Autodesk Inventor part; units mm, degrees
ref_plane "YZ Plane" through (0, 0, 0) normal (1, 0, 0) x (0, 1, 0)
ref_plane "XZ Plane" through (0, 0, 0) normal (0, 1, 0) x (-1, 0, 0)
ref_plane "XY Plane" through (0, 0, 0) normal (0, 0, 1) x (1, 0, 0)
sketch "Sketch1" plane through (0, 0, 0) normal (0, 1, 0) x (-1, 0, 0)
  line L0 (0, 0) -> (0, 12.8)
  line L1 (0, 12.8) -> (-2, 12.8)
  line L2 (-2, 12.8) -> (-2, 7.8)
  line L3 (-2, 7.8) -> (-3, 7.8)
  line L4 (-3, 7.8) -> (-3, 2.8)
  line L5 (-3, 2.8) -> (-5, 2.8)
  line L6 (-5, 2.8) -> (-5, 0)
  line L7 (-5, 0) -> (0, 0)
  dimension "d0" = 10
  dimension "d1" = 6
  dimension "d2" = 4
  dimension "d3" = 5
  dimension "d4" = 5
  dimension "d5" = 2.8
revolve "Revolution1" add sketch "Sketch1" angle 360 about axis through (0, 0, 0) along (0, 0, 1)
thread "Thread1"
sketch "Sketch2" plane through (0, 0, 0) normal (0, 0, -1) x (-1, 0, 0)
  line L0 (0, 1.4434) -> (1.25, 0.7217)
  line L1 (1.25, 0.7217) -> (1.25, -0.7217)
  line L2 (1.25, -0.7217) -> (0, -1.4434)
  line L3 (0, -1.4434) -> (-1.25, -0.7217)
  line L4 (-1.25, -0.7217) -> (-1.25, 0.7217)
  line L5 (-1.25, 0.7217) -> (0, 1.4434)
  point P0 (0, 0)
  point P1 (0, 0)
  dimension "d9" = 2.5
extrude "Extrusion1" cut sketch "Sketch2" against normal blind 2
chamfer "Chamfer1" distance 0.43 angle 45 1 edges at (-2, 0, 12.8)
properties part number "DBSY4-5-5" material "Stainless Steel AISI 304"
Could you check a few things on this model? Use its own coordinates, in mm. A direction names the side the tool comes from. Give positions to 0.01 mm unless a question says otherwise; leave off trailing zeros. Order: outer loops, then holes, each group sorted by start corner. A loop starts at its lowest first (then second) coordinate and runs counter-clockwise, first axis right, second up.
Item 1: If we section it at B-B, the plane z = 5.5: Write out the boundary of the cut face in (x, y), plus the area to 3 significant figures.
Item 2: If we mould it in two halves opening along Y, with no side actions, what happens to faces 1 (the face through (0, 2, 10)), 2 (the face through (0.616, -1.088, 0.986)), 3 (the face through (0, 0, 12.8))? For each: pulls with the +Y half, pulls with the -Y half, needs draft (parallel to the pull), parting line crosses it, or undercut.
Item 3: If we section it at D-D, the plane z = 11: Write out the boundary of the cut face in (x, y).
Item 4: For faces 4 (the face through (-1.08, 4.88, 1.38)), 5 (the face through (-1.25, 0, 1)), 6 (the face through (3.3, 0.1, 2.8)), which set-ups out of +Z, -Z, +X, -X, +Y, -Y let a thin tool reach every point of the face, with its end or its side?
Item 5: If we section it at C-C, the plane y = -2.25: Write out the boundary of the cut face in (x, z).
Item 6: If we section it at A-A, the plane y = 0: Write out the boundary of the cut face in (x, z), plus the area to 3 significant figures.
Item 7: I need wall thicknesses on line 1 (Z direction, x = 4, y = 0); line 2 (Y direction, x = 0, z = 11.5); line 3 (X direction, y = -4, z = 1.75). Which ranges of each line are inside material? Lowest first, please.
Item 8: I'm going to push flat-ended pins straight in: pin 1 (1 mm diameter, centred on y = -0.5, z = 10, fed in from +X); pin 2 (6 mm diameter, centred on x = -3, z = 7.5, fed in from -Y); pin 3 (4 mm diameter, centred on y = 3, z = 11, fed in from -X). Where does each tip first touch, or does it pass through?
Values:
1. outline: circle Ø6 at (0, 0)
1. area: 28.3 mm2
2. face 1: parting line crosses it
2. face 2: undercut
2. face 3: needs draft
3. outline: circle Ø4 at (0, 0)
4. face 4: +Z, -Z
4. face 5: -Z
4. face 6: +Z
5. outline: (-4.47, 0) - (4.47, 0) - (4.47, 2.8) - (1.98, 2.8) - (1.98, 7.8) - (-1.98, 7.8) - (-1.98, 2.8) - (-4.47, 2.8) - close
6. outline: (-5, 0) - (-1.25, 0) - (-1.25, 2) - (1.25, 2) - (1.25, 0) - (5, 0) - (5, 2.8) - (3, 2.8) - (3, 7.8) - (2, 7.8) - (2, 12.37) - (1.57, 12.8) - (-1.57, 12.8) - (-2, 12.37) - (-2, 7.8) - (-3, 7.8) - (-3, 2.8) - (-5, 2.8) - close
6. area: 72.8 mm2
7. line 1: z = 0 to 2.8
7. line 2: y = -2 to 2
7. line 3: x = -3 to 3
8. pin 1: stops at x = 2
8. pin 2: stops at y = -3
8. pin 3: stops at x = -1.73
